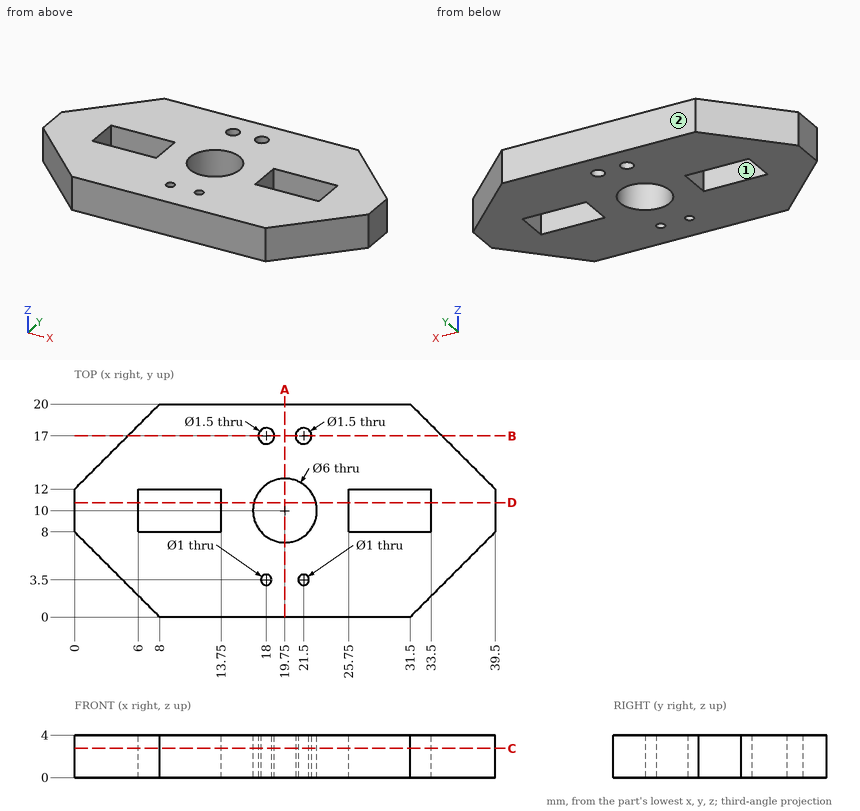
The drawing under review shows one solid part. Ordinate dimensions are in mm from its lowest x, y, z. A direction names the side the tool comes from. Give positions to 0.01 mm unless a question says otherwise; leave off trailing zeros. Order: outer loops, then holes, each group sorted by start corner. A loop starts at its lowest first (then second) coordinate and runs counter-clockwise, first axis right, second up. Notation, with made-up numbers: M 85.5,-3.5 L 144.5,-3.5 A25 ccw 144.5,18.5 Z; hole C 9,2 d5. An arc over 180 degrees is marked long. Answer in a Markdown table with one row per item. Add a question column.
1. For pin 1 Ø3.5 at (x, y) = (19.75, 10) entering from -Z; pin 2 Ø1 at (y, z) = (2.5, 1.5) entering from +X, all flat-tipped, find the tip position at first contact; note any pin that passes through.
2. Machinability: for the marked faces 1 and 2, which of the approach directions +Z, -Z, +X, -X, +Y, -Y give a long, thin tool a straight path to every point of the face, cutting with its end or side? Answer none if there is none.
3. Add section D-D on y = 10.75. State the section outline as (x, z) points, plus the area to 3 significant figures.
4. Add section A-A on x = 19.75. State the section outline as (y, z) points, plus the area to 3 significant figures.
5. Add section C-C on z = 2.75. State the section outline as (x, y) points, plus the area to 3 significant figures.
6. Add section B-B on y = 17. State the section outline as (x, z) points, plus the area to 3 significant figures.
7. To check wall thickness, follow line 1 along X through (y, z) = (10.75, 1.8); line 2 along X through (y, z) = (8.75, 2.3); line 3 along Y through (x, z) = (21.5, 1.4). State the ranges of each line that lie inside material, in increasing order.
The answers:
| question | item | result |
|---|---|---|
| 1 | pin 1 | through |
| 1 | pin 2 | x = 34.5 |
| 2 | face 1 | +Z, -Z |
| 2 | face 2 | +Z, -Z, +X, -X, +Y |
| 3 | outline | M 0,0 L 6,0 L 6,4 L 0,4 Z; M 13.75,0 L 16.85,0 L 16.85,4 L 13.75,4 Z; M 22.65,0 L 25.75,0 L 25.75,4 L 22.65,4 Z; M 33.5,0 L 39.5,0 L 39.5,4 L 33.5,4 Z |
| 3 | area | 72.8 mm2 |
| 4 | outline | M 0,0 L 7,0 L 7,4 L 0,4 Z; M 13,0 L 20,0 L 20,4 L 13,4 Z |
| 4 | area | 56.0 mm2 |
| 5 | outline | M 0,8 L 8,0 L 31.5,0 L 39.5,8 L 39.5,12 L 31.5,20 L 8,20 L 0,12 Z; hole M 6,8 L 13.75,8 L 13.75,12 L 6,12 Z; hole C 19.75,10 d6; hole C 18,17 d1.5; hole C 18,3.5 d1; hole C 21.5,17 d1.5; hole C 21.5,3.5 d1; hole M 25.75,8 L 33.5,8 L 33.5,12 L 25.75,12 Z |
| 5 | area | 567 mm2 |
| 6 | outline | M 5,0 L 17.25,0 L 17.25,4 L 5,4 Z; M 18.75,0 L 20.75,0 L 20.75,4 L 18.75,4 Z; M 22.25,0 L 34.5,0 L 34.5,4 L 22.25,4 Z |
| 6 | area | 106 mm2 |
| 7 | line 1 | 0 to 6, 13.75 to 16.85, 22.65 to 25.75, 33.5 to 39.5 |
| 7 | line 2 | 0 to 6, 13.75 to 17.02, 22.48 to 25.75, 33.5 to 39.5 |
| 7 | line 3 | 0 to 3, 4 to 7.56, 12.44 to 16.25, 17.75 to 20 |
